Autodesk Inventor part; units mm, degrees
ref_plane "YZ Plane" through (0, 0, 0) normal (1, 0, 0) x (0, 1, 0)
ref_plane "XZ Plane" through (0, 0, 0) normal (0, 1, 0) x (-1, 0, 0)
ref_plane "XY Plane" through (0, 0, 0) normal (0, 0, 1) x (1, 0, 0)
sketch "Sketch1" plane through (0, 0, 0) normal (0, 0, 1) x (1, 0, 0)
  arc A0 (-33, 0) -> (33, 0) centre (0, 0) ccw
  arc A1 (-27, 0) -> (27, 0) centre (0, 0) ccw
  line L0 (-33, 0) -> (-27, 0)
  line L1 (27, 0) -> (33, 0)
  dimension "d0" = 66
  dimension "d1" = 54
extrude "Extrusion1" add sketch "Sketch1" along normal blind 10
sketch "Sketch2" plane through (-33, 0, 0) normal (0, 1, 0) x (1, 0, 0)
  line L0 (6, 0) -> (6, -10)
  line L1 (6, 0) -> (-9, 0)
  line L2 (-9, 0) -> (-9, -10)
  line L3 (-9, -10) -> (6, -10)
  line L4 (6, -10) -> (6, 0)
  line L5 (66, 0) -> (60, 0)
  line L6 (60, 0) -> (75, 0)
  line L7 (75, 0) -> (75, -10)
  line L8 (75, -10) -> (60, -10)
  line L9 (60, -10) -> (60, 0)
  point P0 (33, 0)
  dimension "d4" = 15
extrude "Extrusion2" add sketch "Sketch2" against normal blind 5
sketch "Sketch3" plane through (-27, 0, 10) normal (0, 1, 0) x (1, 0, 0)
  circle A0 centre (-9, 5) radius 1.65
  circle A1 centre (63, 5) radius 1.65
  line L0 (0, 10) -> (-15, 10)
  line L1 (-15, 10) -> (-15, 0)
  line L2 (69, 10) -> (54, 10)
  line L3 (69, 0) -> (69, 10)
  point P0 (27, 10)
  dimension "d7" = 5
  dimension "d8" = 6
  dimension "d9" = 5
  dimension "d10" = 6
  dimension "d11" = 3.3
extrude "Extrusion3" cut sketch "Sketch3" against normal blind 5
sketch "Sketch4" plane through (0, 0, 10) normal (0, 0, 1) x (1, 0, 0)
  arc A0 (-33, 0) -> (33, 0) centre (0, 0) ccw
  arc A1 (-20, 0) -> (20, 0) centre (0, 0) ccw
  line L0 (-27, 0) -> (-42, 0)
  line L1 (33, 0) -> (20, 0)
  line L2 (-20, 0) -> (-33, 0)
  dimension "d14" = 40
  dimension "d15" = 66
extrude "Extrusion4" add sketch "Sketch4" along normal blind 5
properties part number "22010B_Tube End Support_V1" material "ABS Plastic"
Here's how the part is built. I have some questions about the finished solid (model axes, mm). A direction names the side the tool comes from. Coordinates: 2 decimals unless noted, no trailing zeros. Write each loop counter-clockwise with the first axis right and the second up, starting at its lowest first coordinate (ties: lowest second). Pieces come first, ordered by that corner, then holes. Notation, with made-up numbers: (41.5, 6) - (55.5, 6) arc R22 ccw to (55.5, 41) - close; hole circle Ø5 at (83.5, 29.25). An arc over 180 degrees is marked (long way). One line per item, written item: value.
1) Suppose I cut it at A-A on x = -36. Write out the boundary of the cut face in (y, z), and give its area (3 significant figures).
Model answer:
outline: (-5, 0) - (0, 0) - (0, 3.35) - (-5, 3.35) - close; (-5, 6.65) - (0, 6.65) - (0, 10) - (-5, 10) - close
area: 33.5 mm²
2) Suppose I cut it at D-D on y = -24. Write out the boundary of the cut face in (x, z), and give its area (3 significant figures).
Model answer:
outline: (-22.65, 0) - (-12.37, 0) - (-12.37, 10) - (12.37, 10) - (12.37, 0) - (22.65, 0) - (22.65, 15) - (-22.65, 15) - close
area: 432 mm²
3) I'm going to push flat-ended pins straight in: P1, Ø5.5, axis at x = 38.5, y = -3.5, coming from the +Z side; P2, Ø8, axis at x = 4.5, y = -16.5, coming from the -Z side; P3, Ø5.5, axis at x = -35, y = -3, coming from the +Z side; P4, Ø4.5, axis at x = 37.5, z = 2.5, coming from the -Y side. Where does each tip first touch, or does it pass through?
Model answer:
P1: stops at z = 10
P2: stops at z = 10
P3: stops at z = 15
P4: stops at y = -5
4) We'd pull the mould along X, two halves only. Please class faces 1 (the cylindrical face through (0.73, -32.99, 7.4)), 2 (the cylindrical face through (0, -20, 12)), 3 (the flat face through (-37, -2, 10)), 4 (the flat face through (-42, -2, 5)): pulls with the +X half, pulls with the -X half, needs draft (parallel to the pull), parting line crosses it, or undercut.
Model answer:
face 1: parting line crosses it
face 2: undercut
face 3: needs draft
face 4: pulls with the -X half
5) Suppose I cut it at B-B on y = -2.5. Write out the boundary of the cut face in (x, z), and give its area (3 significant figures).
Model answer:
outline: (-42, 0) - (-26.88, 0) - (-26.88, 10) - (-19.84, 10) - (-19.84, 15) - (-32.91, 15) - (-32.91, 10) - (-42, 10) - close; (19.84, 10) - (26.88, 10) - (26.88, 0) - (42, 0) - (42, 10) - (32.91, 10) - (32.91, 15) - (19.84, 15) - close; hole circle Ø3.3 at (-36, 5); hole circle Ø3.3 at (36, 5)
area: 416 mm²
6) On a 3-axis mill with a long thin cutter (end or side, diameter ignored), from which of +Z, -Z, +X, -X, +Y, -Y can I reach the whole of each face in a straight line? I mean faces 5 (the flat face through (-38, -5, 5)), 6 (the flat face through (0, -22, 10)), 7 (the flat face through (31, 0, 7)), 8 (the flat face through (38, -5, 5)). Say none if no direction works.
Model answer:
face 5: +Z, -Z, -X, -Y
face 6: -Z, +Y
face 7: +Z, -Z, +X, -X, +Y
face 8: +Z, -Z, +X, -Y
7) I need wall thicknesses on line 1 along Z through (x, y) = (-36, -1); line 2 along X through (y, z) = (-1.25, 5); line 3 along X through (y, z) = (-1.7, 5). Which ranges of each line are inside material? Lowest first, please.
Model answer:
line 1: z = 0 to 3.35, 6.65 to 10
line 2: x = -42 to -37.65, -34.35 to -26.97, 26.97 to 34.35, 37.65 to 42
line 3: x = -42 to -37.65, -34.35 to -26.95, 26.95 to 34.35, 37.65 to 42
8) Suppose I cut it at C-C on x = 0. Write out the boundary of the cut face in (y, z).
Model answer:
outline: (-33, 0) - (-27, 0) - (-27, 10) - (-20, 10) - (-20, 15) - (-33, 15) - close
